Input: part model. Units: mm. Frame: model coordinates. A direction names the side the tool comes from. Give positions to 0.01 mm unless a question says otherwise; leave off trailing zeros. Write each loop counter-clockwise with the first axis right and the second up, starting at its lowest first coordinate (ties: lowest second). Pieces come first, ordered by that corner, then holes. Notation, with made-up numbers: (-1.5, 52.5) -> (25.5, 52.5) arc R16 cw to (25.5, 83.5) -> close; hole circle Ø8 at (-28, 20.5). An arc over 180 degrees is marked (long way). Return JSON: item names as keys, results as strings. Group by question number.
Item 1: Set-up query: faces 4 (the face through (3.39, -1.23, 1.07)), 5 (the face through (-4.31, 3.131, -2.535)), 6 (the face through (-0.5, 3.1, 4.5)). Return all of +Z, -Z, +X, -X, +Y, -Y with unobstructed straight access to the full face (end or side cutting, diameter ignored); none if empty.
Item 2: Line query: line 1 (Z direction, x = -1.25, y = 5.25); line 2 (X direction, y = -0.5, z = -0.5); line 3 (Y direction, x = 3, z = -2.5). Output: solid intervals per line, ascending. Write a range as [from, to].
Item 3: Section B-B, the plane z = -1.5. Return loops of the section in (x, y).
Item 4: Section C-C, the plane x = 0.75. Return loops of the section in (y, z).
Item 5: Mould query, pull axis X, two halves, no side actions, for faces 1 (the face through (2.65, 6.19, 4.63)), 2 (the face through (0.5, 3.1, 4.5)), 3 (the face through (0, -2.5, -2)). Classes: released by +X, released by -X, zero draft, split by the parting line, or undercut.
Item 6: Section D-D, the plane z = -3. Return loops of the section in (x, y), then the cut area to 3 significant figures.
Item 7: Pin query (flat end, axial travel): P1, Ø3, axis at x = -0.5, z = 2, coming from the -Y side; P2, Ø1.5, axis at y = 0.5, z = -2.5, coming from the +X side; P3, Ø1, axis at y = 2.5, z = 3, coming from the +X side; P4, Ø4.5, axis at x = 0, z = 0.79, coming from the -Y side. Return the tip coordinate at first contact, or that it passes through.
Item 8: Section A-A, the plane y = 2.5. Return loops of the section in (x, z), then the cut area to 3 significant figures.
from build123d import *

# Parameters (mm, degrees)
BOSS_EXTRUDE1_DEPTH = 6.35
SKETCH3_R           = 3.555
BOSS_EXTRUDE3_DEPTH = 2.5
SKETCH4_R           = 2.5
CUT_EXTRUDE1_DEPTH  = 9.85
CUT_EXTRUDE2_DEPTH  = 7.35


with BuildPart() as part:
    # Sketch1 → Boss-Extrude1 (new body)
    with BuildSketch(Plane(origin=(0, 0, 0), x_dir=(1, 0, 0), z_dir=(0, 1, 0))):
        Polygon((5.773502692, 0), (2.886751346, 5), (-2.886751346, 5), (-5.773502692, 0), (-2.886751346, -5), (2.886751346, -5), align=None)
    extrude(amount=BOSS_EXTRUDE1_DEPTH)

    # Sketch3 → Boss-Extrude3 (add)
    with BuildSketch(Plane.XZ):
        Circle(SKETCH3_R)
    extrude(amount=BOSS_EXTRUDE3_DEPTH)

    # Sketch4 → Cut-Extrude1 (cut, through all)
    with BuildSketch(Plane(origin=(0, 6.35, 0), x_dir=(1, 0, 0), z_dir=(0, 1, 0))):
        with Locations((0, -0.79)):
            Circle(SKETCH4_R)
    extrude(amount=-CUT_EXTRUDE1_DEPTH, mode=Mode.SUBTRACT)

    # Sketch5 → Cut-Extrude2 (cut, through all)
    with BuildSketch(Plane(origin=(0, 0, 0), x_dir=(-1, 0, 0), z_dir=(0, -1, 0))):
        Polygon((-1, -5), (1, -5), (0, -4), align=None)
    extrude(amount=-CUT_EXTRUDE2_DEPTH, mode=Mode.SUBTRACT)

    # Sketch6 → Cut-Revolve1 (revolve, cut)
    with BuildSketch(Plane.XY):
        Polygon((5.173502692, 6.35), (5.773502692, 6.35), (5.773502692, 5.75), align=None)
        Polygon((5.773502692, 0.6), (5.173502692, 0), (5.773502692, 0), align=None)
    revolve(axis=Axis((0, 0, 0), (0, 1, 0)), mode=Mode.SUBTRACT)


solid = part.part
Answer below:
{
 "1": {"face 4": "-Y", "face 5": "-Z, -X, +Y, -Y", "face 6": "+Z, +Y, -Y"},
 "2": {"line 1": "z = [-5, -1.38], [2.96, 5]", "line 2": "x = [-3.52, -2.14], [2.14, 3.52]", "line 3": "y = [0, 6.35]"},
 "3": {"outline": "(-4.91, 0) -> (-3.22, 0) -> (-3.22, -2.5) -> (-1, -2.5) -> (-1, 6.35) -> (-4.91, 6.35) -> close; (1, -2.5) -> (3.22, -2.5) -> (3.22, 0) -> (4.91, 0) -> (4.91, 6.35) -> (1, 6.35) -> close"},
 "4": {"outline": "(-2.5, -3.47) -> (0, -3.47) -> (0, -5) -> (6.35, -5) -> (6.35, -1.59) -> (-2.5, -1.59) -> close; (-2.5, 3.17) -> (6.35, 3.17) -> (6.35, 4.75) -> (0, 4.75) -> (0, 3.47) -> (-2.5, 3.47) -> close"},
 "5": {"face 1": "released by +X", "face 2": "undercut", "face 3": "zero draft"},
 "6": {"outline": "(-4.04, 0) -> (-1.91, 0) -> (-1.91, -2.5) -> (1.91, -2.5) -> (1.91, 0) -> (4.04, 0) -> (4.04, 6.35) -> (-4.04, 6.35) -> close", "area": "60.9 mm2"},
 "7": {"P1": "stops at y = -2.5", "P2": "stops at x = 4.76", "P3": "stops at x = 4.33", "P4": "passes through"},
 "8": {"outline": "(-5.77, 0) -> (-2.89, -5) -> (2.89, -5) -> (5.77, 0) -> (2.89, 5) -> (1, 5) -> (0, 4) -> (-1, 5) -> (-2.89, 5) -> close; hole circle Ø5 at (0, 0.79)", "area": "66.0 mm2"}
}
